```python
from build123d import *

# Parameters (mm, degrees)
F0_W      = 114
F0_H      = 55
F1_DEPTH  = 10
F2_R      = 6.5183766184
F3_R      = 3
F4_R      = 2.8970562748
F5_R      = 1.7337923038
F6_DEPTH  = 0.5
F7_W      = 14.7860310972
F7_H      = 1.384280622
F8_DEPTH  = 0.5
F9_R      = 4.3601608972
F10_DEPTH = 1.5
F11_W     = 1.1572175405
F11_H     = 12.150795199
F12_DEPTH = 0.4
F13_W     = 81.5876945853
F13_H     = 42.6051579416
F14_DEPTH = 0.5
F16_DEPTH = 0.4
F17_R     = 1.5038769237
F18_DEPTH = 10
F19_W     = 8.4370337427
F19_H     = 1.285196282
F20_DEPTH = 0.5


with BuildPart() as f1:
    # F0 (on Top) → F1 (new body)
    with BuildSketch(Plane.XY):
        Rectangle(F0_W, F0_H)
    extrude(amount=F1_DEPTH)

    # F2
    f2_edges = [f1.edges().sort_by_distance(p)[0] for p in [
        (57, -27.5, 5),
        (-57, -27.5, 5),
        (57, 27.5, 5),
        (-57, 27.5, 5),
    ]]
    fillet(f2_edges, radius=F2_R)

    # F3
    f3_edges = [f1.edges().sort_by_distance(p)[0] for p in [
        (55.090812, -25.590812, 0),
        (-55.090812, -25.590812, 0),
        (-55.090812, 25.590812, 0),
        (55.090812, 25.590812, 0),
    ]]
    fillet(f3_edges, radius=F3_R)

    # F4
    f4_edges = [f1.edges().sort_by_distance(p)[0] for p in [
        (0, 27.5, 10),
        (55.090812, 25.590812, 10),
        (-55.090812, 25.590812, 10),
        (57, 0, 10),
        (-57, 0, 10),
        (55.090812, -25.590812, 10),
        (-55.090812, -25.590812, 10),
        (0, -27.5, 10),
    ]]
    fillet(f4_edges, radius=F4_R)

    # F5 (on face) → F6 (join)
    with BuildSketch(Plane(origin=(0, 27.5, 0), x_dir=(-1, 0, 0), z_dir=(0, 1, 0))):
        with Locations((0, 4.9682608806)):
            Circle(F5_R)
    extrude(amount=F6_DEPTH)

    # F7 (on face) → F8 (join)
    with BuildSketch(Plane(origin=(0, 27.5, 0), x_dir=(-1, 0, 0), z_dir=(0, 1, 0))):
        with Locations((19.3366743624, 5.336954724)):
            Rectangle(F7_W, F7_H)
    extrude(amount=F8_DEPTH)

    # F9 (on face) → F10 (cut)
    with BuildSketch(Plane(origin=(0, 0, 0), x_dir=(1, 0, 0), z_dir=(0, 0, -1))):
        with Locations((-41.5013991296, 0)):
            Circle(F9_R)
    extrude(amount=-F10_DEPTH, mode=Mode.SUBTRACT)

    # F11 (on face) → F12 (cut)
    with BuildSketch(Plane.XY.offset(10)):
        with Locations((-51.5272360634, 0)):
            Rectangle(F11_W, F11_H)
    extrude(amount=-F12_DEPTH, mode=Mode.SUBTRACT)

    # F13 (on face) → F14 (cut)
    with BuildSketch(Plane.XY.offset(10)):
        Rectangle(F13_W, F13_H)
    extrude(amount=-F14_DEPTH, mode=Mode.SUBTRACT)

    # F15 (on face) → F16 (cut)
    with BuildSketch(Plane.XZ.offset(27.5)):
        Polygon((-41.7614616454, 6.1881397851), (-44.9712947011, 6.1881397851), (-45.7120239735, 5.5502885953), (-45.7120239735, 4.459768068), (-41.1441847682, 4.459768068), (-41.1441847682, 5.5502885953), align=None)
    extrude(amount=-F16_DEPTH, mode=Mode.SUBTRACT)

    # F17 (on face) → F18 (cut)
    with BuildSketch(Plane(origin=(-57, 0, 0), x_dir=(0, -1, 0), z_dir=(-1, 0, 0))):
        with Locations((13.8453152031, 4.8393858597)):
            Circle(F17_R)
    extrude(amount=-F18_DEPTH, mode=Mode.SUBTRACT)

    # F19 (on face) → F20 (join)
    with BuildSketch(Plane(origin=(-57, 0, 0), x_dir=(0, -1, 0), z_dir=(-1, 0, 0))):
        with Locations((-14.7477723658, 4.9256444909)):
            Rectangle(F19_W, F19_H)
    extrude(amount=F20_DEPTH)


solid = f1.part
```
CAD build for the part. Positions are in the model's coordinates, mm. A direction names the side the tool comes from. Give positions to 0.01 mm unless a question says otherwise; leave off trailing zeros. Order: outer loops, then holes, each group sorted by start corner. A loop starts at its lowest first (then second) coordinate and runs counter-clockwise, first axis right, second up.
(1) Tool access for faces 1 (the cylindrical face through (-55.14, -25.54, 5.08)), 2 (the cylindrical face through (0.7, 26.6, 9.2)), 3 (the cylindrical face through (-37.474, 1.67, 0.74)), 4 (the cylindrical face through (-52.07, -14.539, 3.505)), 5 (the cylindrical face through (-0.93, 27.75, 6.43)): list every direction of +Z, -Z, +X, -X, +Y, -Y with a clear straight run to the whole face (end or side of a thin tool).
(2) Saw through at B-B, the plane y = 0. Give the cut face in (x, z), then the cut area to 3 significant figures.
(3) Saw through at C-C, the plane x = 0. Give the cut face in (y, z).
(4) Saw through at D-D, the plane y = 15. Give the cut face in (x, z).
(5) Saw through at A-A, the plane x = 47. Give the cut face in (y, z).
(6) Drill centre lines: L1, parallel to Z at x = -5, y = 12; L2, parallel to Y at x = -4.5, z = 3; L3, parallel to X at y = -1.5, z = 7.25. Where is each one in solid material? Low to high.
(7) Flat gauge pins, fed straight in: pin 1 (0.6 mm diameter, centred on y = 10.5, z = 9.5, fed in from +X); pin 2 (1.5 mm diameter, centred on x = -15, y = 14.5, fed in from +Z); pin 3 (2 mm diameter, centred on x = -43, z = 4.5, fed in from +Y). Where does each tip first touch, or does it go through?
(8) Mould opens along Z. For faces 6 (the flat face through (-47, -14, 5)), 7 (the cylindrical face through (-55.14, 25.54, 5.08)), 8 (the flat face through (-1, -22, 10)) say: released by +Z, released by -Z, zero draft, split by the parting line, or undercut.
Results found:
1. face 1: +Z, -Z, -X, -Y
1. face 2: +Z, +X, -X, +Y
1. face 3: -Z
1. face 4: -X
1. face 5: +Y
2. outline: (-57, 3) arc R3 ccw to (-54, 0) - (-45.86, 0) - (-45.86, 1.5) - (-37.14, 1.5) - (-37.14, 0) - (54, 0) arc R3 ccw to (57, 3) - (57, 7.1) arc R2.9 ccw to (54.1, 10) - (40.79, 10) - (40.79, 9.5) - (-40.79, 9.5) - (-40.79, 10) - (-50.95, 10) - (-50.95, 9.6) - (-52.11, 9.6) - (-52.11, 10) - (-54.1, 10) arc R2.9 ccw to (-57, 7.1) - close
2. area: 1,080 mm2
3. outline: (-27.5, 3) arc R3 ccw to (-24.5, 0) - (24.5, 0) arc R3 ccw to (27.5, 3) - (27.5, 3.23) - (28, 3.23) - (28, 6.7) - (27.5, 6.7) - (27.5, 7.1) arc R2.9 ccw to (24.6, 10) - (21.3, 10) - (21.3, 9.5) - (-21.3, 9.5) - (-21.3, 10) - (-24.6, 10) arc R2.9 ccw to (-27.5, 7.1) - close
4. outline: (-57.5, 4.28) - (-57, 4.28) - (-57, 3) arc R3 ccw to (-54, 0) - (54, 0) arc R3 ccw to (57, 3) - (57, 7.1) arc R2.9 ccw to (54.1, 10) - (40.79, 10) - (40.79, 9.5) - (-40.79, 9.5) - (-40.79, 10) - (-54.1, 10) arc R2.9 ccw to (-57, 7.1) - (-57, 5.57) - (-57.5, 5.57) - close
5. outline: (-27.5, 3) arc R3 ccw to (-24.5, 0) - (24.5, 0) arc R3 ccw to (27.5, 3) - (27.5, 7.1) arc R2.9 ccw to (24.6, 10) - (-24.6, 10) arc R2.9 ccw to (-27.5, 7.1) - close
6. L1: z = 0 to 9.5
6. L2: y = -27.5 to 27.5
6. L3: x = -57 to 57
7. pin 1: stops at x = 56.1
7. pin 2: stops at z = 9.5
7. pin 3: stops at y = 27.5
8. face 6: undercut
8. face 7: zero draft
8. face 8: released by +Z
